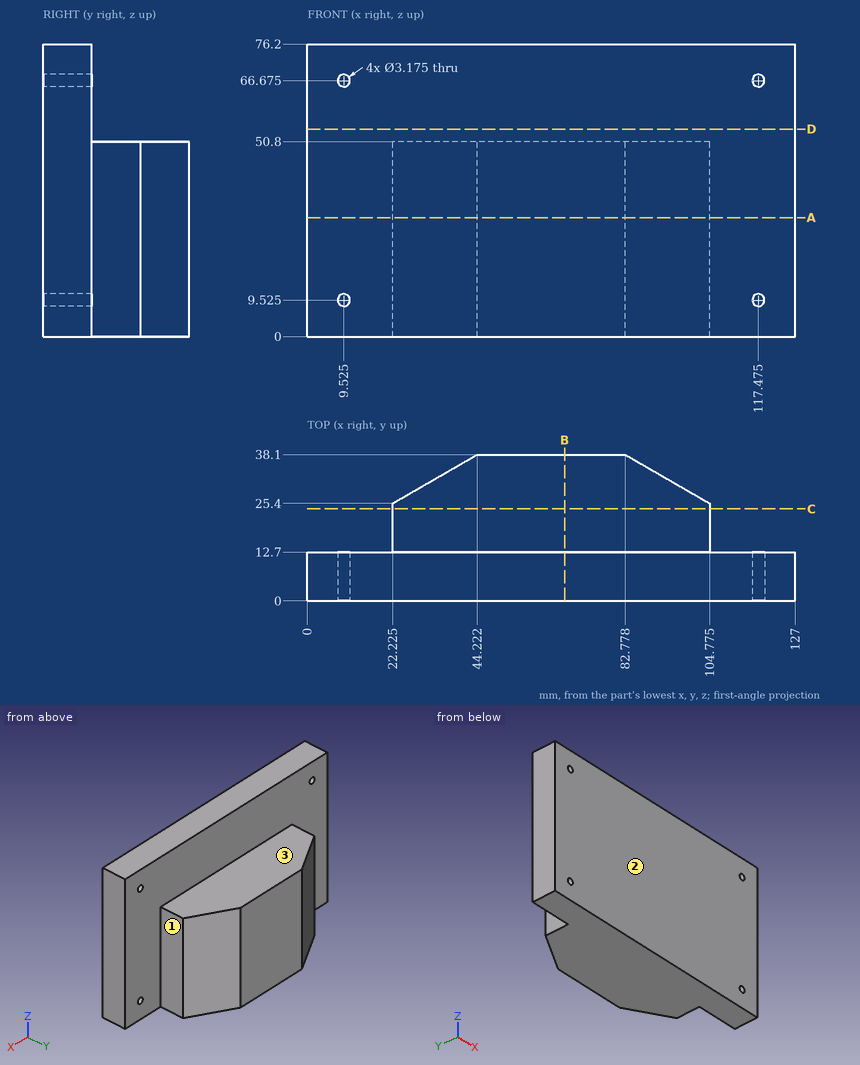
Input: dimensioned drawing with shaded views. Units: mm. Origin: part minimum x, y, z. A direction names the side the tool comes from. Round coordinates to 2 decimals unless told otherwise and drop trailing zeros. Order: outer loops, then holes, each group sorted by start corner. A loop starts at its lowest first (then second) coordinate and runs counter-clockwise, first axis right, second up.
1. Cut plane A-A, the plane z = 31. Output: boundary loops of the cut face in (x, y) (3 decimals), then the cut area to 3 significant figures.
The answers:
outline: (0, 0) - (127, 0) - (127, 12.7) - (104.775, 12.7) - (104.775, 25.4) - (82.778, 38.1) - (44.222, 38.1) - (22.225, 25.4) - (22.225, 12.7) - (0, 12.7) - close
area: 3,430 mm2
2. Cut plane B-B, the plane x = 67. Output: boundary loops of the cut face in (y, z).
The answers:
outline: (0, 0) - (38.1, 0) - (38.1, 50.8) - (12.7, 50.8) - (12.7, 76.2) - (0, 76.2) - close
3. Pin query (flat end, axial travel): P1, Ø6, axis at y = 13, z = 52.5, coming from the +X side; P2, Ø4, axis at y = 21.5, z = 31.5, coming from the +X side (3 decimals); P3, Ø1, axis at y = 21.5, z = 45, coming from the -X side (3 decimals); P4, Ø2, axis at y = 33, z = 47, coming from the +X side. Return the tip coordinate at first contact, or that it passes through.
The answers:
P1: stops at x = 127
P2: stops at x = 104.775
P3: stops at x = 22.225
P4: stops at x = 93.34
4. Material intervals for line 1 (Z direction, x = 77.5, y = 21); line 2 (Y direction, x = 44.5, z = 69); line 3 (X direction, y = 22.5, z = 27.5) (3 decimals), sorted ascending.
The answers:
line 1: z = 0 to 50.8
line 2: y = 0 to 12.7
line 3: x = 22.225 to 104.775
5. Cut plane D-D, the plane z = 54. Output: boundary loops of the cut face in (x, y), then the cut area to 3 significant figures.
The answers:
outline: (0, 0) - (127, 0) - (127, 12.7) - (0, 12.7) - close
area: 1,610 mm2
6. Set-up query: the marked faces 1, 2 and 3. Return all of +Z, -Z, +X, -X, +Y, -Y with unobstructed straight access to the full face (end or side cutting, diameter ignored); none if empty.
The answers:
face 1: +Z, -Z, +X, +Y
face 2: +Z, -Z, +X, -X, -Y
face 3: +Z, +X, -X, +Y
7. Cut plane C-C, the plane y = 24. Output: boundary loops of the cut face in (x, z) (3 decimals).
The answers:
outline: (22.225, 0) - (104.775, 0) - (104.775, 50.8) - (22.225, 50.8) - close
